from build123d import *

# Parameters (mm, degrees)
F1_DEPTH = 4.318
F3_D     = 13.97
F4_W     = 33.02
F4_H     = 20.32
F4_H_2   = 20.409275
F5_DEPTH = 2.54
F8_D     = 4.572
F9_D     = 4.064


with BuildPart() as f1:
    # F0 (on Front) → F1 (new body)
    with BuildSketch(Plane.XZ):
        with BuildLine():
            Line((47.625, 0), (-47.625, 0))
            ThreePointArc((-47.625, 0), (-49.421051, -0.743949), (-50.165, -2.54))
            Line((-50.165, -2.54), (-50.165, -60.96))
            ThreePointArc((-50.165, -60.96), (-49.421051, -62.756051), (-47.625, -63.5))
            Line((-47.625, -63.5), (47.625, -63.5))
            ThreePointArc((47.625, -63.5), (49.421051, -62.756051), (50.165, -60.96))
            Line((50.165, -60.96), (50.165, -2.54))
            ThreePointArc((50.165, -2.54), (49.421051, -0.743949), (47.625, 0))
        make_face()
    extrude(amount=F1_DEPTH)

    # F3 (through all)
    with Locations(Plane.XZ.offset(4.318)):
        with Locations((-21.2598, -29.3116), (21.2598, -29.3116)):
            Hole(F3_D / 2)

    # F4 (on face) → F5 (cut)
    with BuildSketch(Plane.XZ.offset(4.318)):
        with Locations((0, -10.16)):
            Rectangle(F4_W, F4_H)
        with Locations((-33.655, -10.16)):
            Rectangle(F4_W, F4_H)
        with Locations((33.655, -10.204637)):
            Rectangle(F4_W, F4_H_2)
    extrude(amount=-F5_DEPTH, mode=Mode.SUBTRACT)

    # F8 (through all)
    with Locations(Plane(origin=(0, 0, 0), x_dir=(-1, 0, 0), z_dir=(0, 1, 0))):
        with Locations((-23.9268, -60.198), (23.9268, -60.198)):
            Hole(F8_D / 2)

    # F9 (through all)
    with Locations(Plane(origin=(0, 0, 0), x_dir=(-1, 0, 0), z_dir=(0, 1, 0))):
        with Locations((-14.4018, -58.547), (14.4018, -58.547)):
            Hole(F9_D / 2)


solid = f1.part
CAD build for the part. Positions are in the model's coordinates, mm. A direction names the side the tool comes from. Give positions to 0.01 mm unless a question says otherwise; leave off trailing zeros. Write each loop counter-clockwise with the first axis right and the second up, starting at its lowest first coordinate (ties: lowest second). Pieces come first, ordered by that corner, then holes. Notation, with made-up numbers: (87.5, 60) -> (92.5, 60) arc R14 cw to (92.5, 77) -> close; hole circle Ø3 at (45, 42.5). An arc over 180 degrees is marked (long way). Return JSON: item names as keys, results as strings.
Item 1: Tool access for faces 4 (the flat face through (0, -1.778, -10)), 5 (the flat face through (-17.145, -3, -10)), 6 (the flat face through (33, -3, -20.409)): list every direction of +Z, -Z, +X, -X, +Y, -Y with a clear straight run to the whole face (end or side of a thin tool).
Answer below:
{"face 4": "+Z, -Y", "face 5": "+Z, -X, -Y", "face 6": "+Z, +X, -Y"}
Item 2: Two-plate mould, pull along Z, no slides. Class faces 1 (the flat face through (16.51, -3, -10)), 2 (the flat face through (-34, -3, -20.32)), 3 (the cylindrical face through (26.107, -2.189, -59.511)): +Z half, -Z half, draft (parallel to the pull), parting line (faces both ways), or undercut.
Answer below:
{"face 1": "draft", "face 2": "+Z half", "face 3": "undercut"}
Item 3: Band-saw the part on B-B (x = 10). List the corners of the cut face in (y, z), then the cut area to 3 significant figures.
Answer below:
{"outline": "(-4.32, -63.5) -> (0, -63.5) -> (0, 0) -> (-1.78, 0) -> (-1.78, -20.32) -> (-4.32, -20.32) -> close", "area": "223 mm2"}
Item 4: Drop flat-ended pins along their axis: pin 1 (0.8 mm diameter, centred on y = -3.5, z = -12, fed in from -X) (3 decimals); pin 2 (6 mm diameter, centred on x = 23.93, z = -60.2, fed in from -Y); pin 3 (6 mm diameter, centred on x = 30, z = -11.5, fed in from -Y); pin 4 (0.8 mm diameter, centred on y = -3.5, z = -14, fed in from +X) (3 decimals). Give the stop position or say it passes through.
Answer below:
{"pin 1": "stops at x = -17.145", "pin 2": "stops at y = -4.32", "pin 3": "stops at y = -1.78", "pin 4": "stops at x = 17.145"}
Item 5: Band-saw the part on A-A (z = -28). List the corners of the cut face in (x, y) (3 decimals).
Answer below:
{"outline": "(-50.165, -4.318) -> (-28.121, -4.318) -> (-28.121, 0) -> (-50.165, 0) -> close; (-14.399, -4.318) -> (14.399, -4.318) -> (14.399, 0) -> (-14.399, 0) -> close; (28.121, -4.318) -> (50.165, -4.318) -> (50.165, 0) -> (28.121, 0) -> close"}
Item 6: Band-saw the part on D-D (y = -2.85). List the corners of the cut face in (x, z) (3 decimals), then the cut area to 3 significant figures.
Answer below:
{"outline": "(-50.165, -60.96) arc R2.54 ccw to (-47.625, -63.5) -> (47.625, -63.5) arc R2.54 ccw to (50.165, -60.96) -> (50.165, -20.409) -> (17.145, -20.409) -> (17.145, 0) -> (16.51, 0) -> (16.51, -20.32) -> (-16.51, -20.32) -> (-16.51, 0) -> (-17.145, 0) -> (-17.145, -20.32) -> (-50.165, -20.32) -> close; hole circle Ø13.97 at (-21.26, -29.312); hole circle Ø4.572 at (-23.927, -60.198); hole circle Ø4.064 at (-14.402, -58.547); hole circle Ø4.064 at (14.402, -58.547); hole circle Ø13.97 at (21.26, -29.312); hole circle Ø4.572 at (23.927, -60.198)", "area": "3,990 mm2"}
Item 7: Band-saw the part on C-C (z = -6). List the corners of the cut face in (x, y) (3 decimals), then the cut area to 3 significant figures.
Answer below:
{"outline": "(-50.165, -1.778) -> (-17.145, -1.778) -> (-17.145, -4.318) -> (-16.51, -4.318) -> (-16.51, -1.778) -> (16.51, -1.778) -> (16.51, -4.318) -> (17.145, -4.318) -> (17.145, -1.778) -> (50.165, -1.778) -> (50.165, 0) -> (-50.165, 0) -> close", "area": "182 mm2"}
Item 8: Drill centre lines: probe 1 along X at (y, z) = (-3.4, -58.5) (3 decimals); probe 2 along X at (y, z) = (-2.1, -34.5) (3 decimals); probe 3 along Z at (x, y) = (25, -1.6). Where is each one in solid material? Low to high.
Answer below:
{"probe 1": "x = -50.165 to -25.457, -22.396 to -16.433, -12.37 to 12.37, 16.433 to 22.396, 25.457 to 50.165", "probe 2": "x = -50.165 to -25.936, -16.583 to 16.583, 25.936 to 50.165", "probe 3": "z = -63.5 to -62.22, -58.18 to -35.21, -23.41 to 0"}
